Read the model definition and answer for the solid it produces. Units are mm, in the model's axes. Face numbers are marked on the shaded views. A direction names the side the tool comes from. Round coordinates to 2 decimals unless told otherwise and drop trailing zeros. Loops run counter-clockwise (first coordinate to the right, second up) from the corner with the lowest first, then second, coordinate; pieces in that order, holes last. Notation, with made-up numbers: M -19,9 L 31,9 A31 cw 31,43 Z; hole C 1,59 d10. An arc over 180 degrees is marked long. Write each question's results on one line, items separated by ' | '.
```python
from build123d import *

# Parameters (mm, degrees)
F1_DEPTH = 10
F2_DEPTH = 12
F3_SIZE  = 5
F4_SIZE  = 1.99999
F5_R     = 7.5
F6_DEPTH = 5
F7_R     = 4.99999
F9_DEPTH = 9


# Not quite as in the source:
# - a fillet or chamfer is up to 0.001 mm smaller than in the source, because OpenCascade refuses the exact size
# - a feature names something its author has since deleted; it is built from what else it names


with BuildPart() as f1:
    # F0 (on Right) → F1 (new body)
    with BuildSketch(Plane.YZ):
        with BuildLine():
            Line((11.25, 3.75), (20.2777587519, 9.75))
            ThreePointArc((20.2777587519, 9.75), (15.9099025767, 15.9099025767), (9.75, 20.2777587519))
            Line((9.75, 20.2777587519), (3.75, 11.25))
            Line((3.75, 11.25), (0, 11.25))
            Line((0, 11.25), (-3.75, 11.25))
            Line((-3.75, 11.25), (-9.75, 20.2777587519))
            ThreePointArc((-9.75, 20.2777587519), (-15.9099025767, 15.9099025767), (-20.2777587519, 9.75))
            Line((-20.2777587519, 9.75), (-11.25, 3.75))
            Line((-11.25, 3.75), (-11.25, 0))
            Line((-11.25, 0), (-11.25, -3.75))
            Line((-11.25, -3.75), (-20.2777587519, -9.75))
            ThreePointArc((-20.2777587519, -9.75), (-15.9099025767, -15.9099025767), (-9.75, -20.2777587519))
            Line((-9.75, -20.2777587519), (-3.75, -11.25))
            Line((-3.75, -11.25), (0, -11.25))
            Line((0, -11.25), (3.75, -11.25))
            Line((3.75, -11.25), (9.75, -20.2777587519))
            ThreePointArc((9.75, -20.2777587519), (15.9099025767, -15.9099025767), (20.2777587519, -9.75))
            Line((20.2777587519, -9.75), (11.25, -3.75))
            Line((11.25, -3.75), (11.25, 0))
            Line((11.25, 0), (11.25, 3.75))
        make_face()
    extrude(amount=F1_DEPTH)

    # F0 (on Right) → F2 (join)
    with BuildSketch(Plane.YZ):
        with BuildLine():
            Line((3.75, 11.25), (9.75, 20.2777587519))
            ThreePointArc((9.75, 20.2777587519), (0, 22.5), (-9.75, 20.2777587519))
            Line((-9.75, 20.2777587519), (-3.75, 11.25))
            Line((-3.75, 11.25), (0, 11.25))
            Line((0, 11.25), (3.75, 11.25))
        make_face()
        with BuildLine():
            ThreePointArc((-9.75, 20.2777587519), (0, 22.5), (9.75, 20.2777587519))
            Line((9.75, 20.2777587519), (6, 25.5))
            Line((6, 25.5), (0, 25.5))
            Line((0, 25.5), (-6, 25.5))
            Line((-6, 25.5), (-9.75, 20.2777587519))
        make_face()
        with BuildLine():
            Line((-11.25, 3.75), (-20.2777587519, 9.75))
            ThreePointArc((-20.2777587519, 9.75), (-22.5, 0), (-20.2777587519, -9.75))
            Line((-20.2777587519, -9.75), (-11.25, -3.75))
            Line((-11.25, -3.75), (-11.25, 0))
            Line((-11.25, 0), (-11.25, 3.75))
        make_face()
        with BuildLine():
            ThreePointArc((-20.2777587519, -9.75), (-22.5, 0), (-20.2777587519, 9.75))
            Line((-20.2777587519, 9.75), (-25.5, 6))
            Line((-25.5, 6), (-25.5, 0))
            Line((-25.5, 0), (-25.5, -6))
            Line((-25.5, -6), (-20.2777587519, -9.75))
        make_face()
        with BuildLine():
            ThreePointArc((-9.75, -20.2777587519), (0, -22.5), (9.75, -20.2777587519))
            Line((9.75, -20.2777587519), (3.75, -11.25))
            Line((3.75, -11.25), (0, -11.25))
            Line((0, -11.25), (-3.75, -11.25))
            Line((-3.75, -11.25), (-9.75, -20.2777587519))
        make_face()
        with BuildLine():
            Line((6, -25.5), (9.75, -20.2777587519))
            ThreePointArc((9.75, -20.2777587519), (0, -22.5), (-9.75, -20.2777587519))
            Line((-9.75, -20.2777587519), (-6, -25.5))
            Line((-6, -25.5), (0, -25.5))
            Line((0, -25.5), (6, -25.5))
        make_face()
        with BuildLine():
            ThreePointArc((20.2777587519, -9.75), (21.93740609, -5.0000214041), (22.5, 0))
            ThreePointArc((22.5, 0), (21.93740609, 5.0000214041), (20.2777587519, 9.75))
            Line((20.2777587519, 9.75), (11.25, 3.75))
            Line((11.25, 3.75), (11.25, 0))
            Line((11.25, 0), (11.25, -3.75))
            Line((11.25, -3.75), (20.2777587519, -9.75))
        make_face()
        with BuildLine():
            ThreePointArc((20.2777587519, 9.75), (21.93740609, 5.0000214041), (22.5, 0))
            ThreePointArc((22.5, 0), (21.93740609, -5.0000214041), (20.2777587519, -9.75))
            Line((20.2777587519, -9.75), (25.5, -6))
            Line((25.5, -6), (25.5, 0))
            Line((25.5, 0), (25.5, 6))
            Line((25.5, 6), (20.2777587519, 9.75))
        make_face()
    extrude(amount=F2_DEPTH)

    # F3
    f3_edges = [f1.edges().sort_by_distance(p)[0] for p in [
        (10, 15.909903, 15.909903),
        (10, -15.909903, 15.909903),
        (10, -15.909903, -15.909903),
        (10, 15.909903, -15.909903),
    ]]
    chamfer(f3_edges, length=F3_SIZE)

    # F4 (size 2 in the source; OpenCascade refuses exactly that, so slightly less here)
    f4_edges = [f1.edges().sort_by_distance(p)[0] for p in [
        (12, 0, 25.5),
        (12, -7.875, 22.888879),
        (12, 7.875, 22.888879),
        (12, -6.75, 15.763879),
        (12, 6.75, 15.763879),
        (12, 0, 11.25),
        (12, -15.763879, 6.75),
        (12, -22.888879, 7.875),
        (12, -25.5, 0),
        (12, -22.888879, -7.875),
        (12, -15.763879, -6.75),
        (12, -11.25, 0),
        (12, 0, -11.25),
        (12, -6.75, -15.763879),
        (12, -7.875, -22.888879),
        (12, 6.75, -15.763879),
        (12, 0, -25.5),
        (12, 7.875, -22.888879),
        (12, 15.763879, -6.75),
        (12, 11.25, 0),
        (12, 15.763879, 6.75),
        (12, 22.888879, 7.875),
        (12, 25.5, 0),
        (12, 22.888879, -7.875),
    ]]
    chamfer(f4_edges, length=F4_SIZE)

    # F5 (on face) → F6 (join)
    with BuildSketch(Plane.YZ.offset(10)):
        Circle(F5_R)
    extrude(amount=F6_DEPTH)

    # F7 (radius 5 in the source; OpenCascade refuses exactly that, so slightly less here)
    f7_edges = [f1.edges().sort_by_distance(p)[0] for p in [
        (15, -7.5, 0),
    ]]
    fillet(f7_edges, radius=F7_R)

    # F8 (on face) → F9 (join)
    with BuildSketch(Plane.YZ):
        with BuildLine():
            ThreePointArc((0, -11.25), (7.9549512883, -7.9549512883), (11.25, 0))
            ThreePointArc((11.25, 0), (7.9549512883, 7.9549512883), (0, 11.25))
            ThreePointArc((0, 11.25), (-7.9549512883, 7.9549512883), (-11.25, 0))
            ThreePointArc((-11.25, 0), (-7.9549512883, -7.9549512883), (0, -11.25))
        make_face()
    extrude(amount=-F9_DEPTH)


solid = f1.part
```
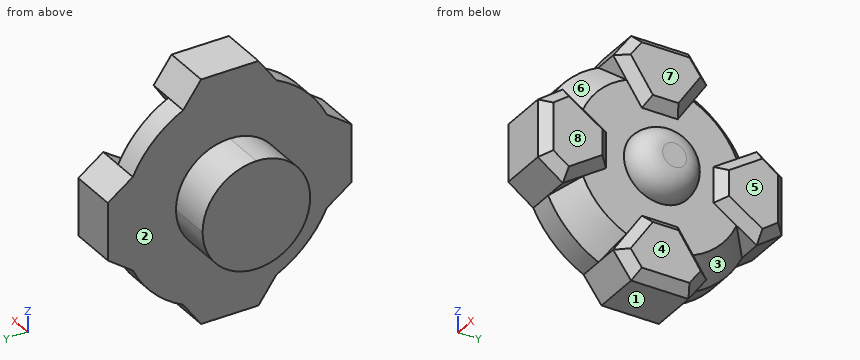
1. Given P1, Ø5, axis at y = 6.5, z = -10.5, coming from the +X side; P2, Ø1.5, axis at y = -14, z = 12, coming from the -X side; P3, Ø3, axis at x = -1, y = -1.5, coming from the +Z side; P4, Ø3, axis at y = 19.5, z = -1.5, coming from the +X side, each flat-ended and moving along its own axis, determine where each tip first touches the part or whether it passes through.
Completed:
P1: stops at x = 10 | P2: stops at x = 0 | P3: stops at z = 25.5 | P4: stops at x = 12
2. Find the intervals of material crossed by L1, parallel to X at y = -11, z = 2.5; L2, parallel to X at y = 20, z = -4.5; L3, parallel to Z at x = 7, y = -13.5, in increasing order.
Completed:
L1: x = 0 to 10 | L2: x = 0 to 12 | L3: z = -15.43 to 15.43
3. Determine the mould class of the marked faces 1, 2 and 3 for opening direction Z: released by +Z, released by -Z, zero draft, split by the parting line, or undercut.
Completed:
face 1: released by -Z | face 2: zero draft | face 3: undercut
4. Find section A-A, the plane y = 21. Give the vertices of the cut face in (x, z).
Completed:
outline: M 0,-9.23 L 10,-9.23 L 12,-6.77 L 12,6.77 L 10,9.23 L 0,9.23 Z
5. Which of the six approach directions +Z, -Z, +X, -X, +Y, -Y give full straight-line access (tool end or side, diameter ignored) to the marked faces 4, 5, 6, 7 and 8?
Completed:
face 4: -Z, +X, +Y, -Y | face 5: +Z, -Z, +X, +Y | face 6: +X | face 7: +Z, +X, +Y, -Y | face 8: +Z, -Z, +X, -Y
6. Find section B-B, the plane x = -3.5. Give the vertices of the cut face in (y, z), then the cut area to 3 significant figures.
Completed:
outline: C 0,0 d22.5 | area: 398 mm2
